Check sheet for the modelled part. Datum: model origin and axes. Units: mm. A direction names the side the tool comes from. Round coordinates to 2 decimals unless told otherwise and drop trailing zeros. Write each loop counter-clockwise with the first axis right and the second up, starting at its lowest first coordinate (ties: lowest second). Pieces come first, ordered by that corner, then holes. Notation, with made-up numbers: (-12.75, 71.25) - (10.25, 71.25) arc R12 cw to (10.25, 77.25) - close; hole circle Ø8 at (-10.75, 57.25). An arc over 180 degrees is marked (long way). Answer as a JSON object with one key per item and string values. Group by question number.
Item 1: Sectioned sample at B-B on z = 8.75. Record the boundary of the cut face in (x, y), plus the area to 3 significant figures.
Item 2: Release check for a two-part mould opening along X. For faces 1 (the cylindrical face through (-40.6, -26.43, 19.26)), 2 (the flat face through (45, 0, 10)), 3 (the cylindrical face through (-26.503, 25.131, 2.465)) record: pulls with the +X half, pulls with the -X half, needs draft (parallel to the pull), parting line crosses it, or undercut.
Item 3: Thickness scan on line 1 (Y direction, x = -24.5, z = 1.15); line 2 (X direction, y = 1.5, z = 12). Record the ranges inside material, lowest first.
Item 4: Sectioned sample at C-C on x = -20.5. Record the boundary of the cut face in (y, z).
Item 5: Set-up check for faces 4 (the cylindrical face through (26.43, -40.6, 19.26)), 5 (the flat face through (-43, 22, 18.5)), 6 (the cylindrical face through (40.6, -17.57, 19.26)), 7 (the cylindrical face through (-35.521, 38.966, 10.14)), 8 (the flat face through (-30, 0, 12)): record each of +Z, -Z, +X, -X, +Y, -Y from which the full face is reachable in a straight line by a thin tool's end or side.
Item 6: Gauge pin test, flat ends, axial feed: P1, Ø0.6, axis at x = -39, z = 20, coming from the +Y side; P2, Ø1.2, axis at x = -44, z = 19.5, coming from the -Y side; P3, Ø6.5, axis at x = -24.5, y = 24.5, coming from the +Z side. Record the tip position at first contact, or that the pin passes through.
Item 7: Sectioned sample at D-D on y = -36.5. Record the boundary of the cut face in (x, z), plus the area to 3 significant figures.
Item 8: Sectioned sample at A-A on y = 10.5. Record the boundary of the cut face in (x, z), plus the area to 3 significant figures.
```python
from build123d import *

# Parameters (mm, degrees)
ESQUISSE1_W             = 90
ESQUISSE1_H             = 90
BOSS_EXTRU_1_DEPTH      = 20
ENL_V_MAT_EXTRU_1_DEPTH = 15
ENL_V_MAT_EXTRU_2_DEPTH = 0.5
CONG_1_R                = 10
ESQUISSE6_R             = 4
ENL_V_MAT_EXTRU_4_DEPTH = 21
ESQUISSE7_R             = 5
ENL_V_MAT_EXTRU_5_DEPTH = 6
ENL_V_MAT_EXTRU_6_DEPTH = 1.5
TROU_TARAUD_M51_D       = 4.2
TROU_TARAUD_M51_DEPTH   = 14
TROU_TARAUD_M51_TIP     = 1.2618073
ENL_V_MAT_EXTRU_7_REACH = 92
ESQUISSE4_R             = 7.75


with BuildPart() as part:
    # Esquisse1 → Boss.-Extru.1 (new body)
    with BuildSketch(Plane.XY):
        Rectangle(ESQUISSE1_W, ESQUISSE1_H)
    extrude(amount=BOSS_EXTRU_1_DEPTH)

    # Esquisse2 → Enlèv. mat.-Extru.1 (cut)
    with BuildSketch(Plane.XY.offset(20)):
        with BuildLine():
            Line((-25, -30), (25, -30))
            ThreePointArc((25, -30), (28.535533906, -28.535533906), (30, -25))
            Line((30, -25), (30, 25))
            ThreePointArc((30, 25), (28.535533906, 28.535533906), (25, 30))
            Line((25, 30), (-25, 30))
            ThreePointArc((-25, 30), (-28.535533906, 28.535533906), (-30, 25))
            Line((-30, 25), (-30, -25))
            ThreePointArc((-30, -25), (-28.535533906, -28.535533906), (-25, -30))
        make_face()
    extrude(amount=-ENL_V_MAT_EXTRU_1_DEPTH, mode=Mode.SUBTRACT)

    # Esquisse3 → Enlèv. mat.-Extru.2 (cut)
    with BuildSketch(Plane.XY.offset(20)):
        with BuildLine():
            Line((25, 32), (12, 32))
            ThreePointArc((12, 32), (10.585786438, 31.414213562), (10, 30))
            Line((10, 30), (25, 30))
            ThreePointArc((25, 30), (28.535533906, 28.535533906), (30, 25))
            Line((30, 25), (30, -25))
            ThreePointArc((30, -25), (28.535533906, -28.535533906), (25, -30))
            Line((25, -30), (-25, -30))
            ThreePointArc((-25, -30), (-28.535533906, -28.535533906), (-30, -25))
            Line((-30, -25), (-30, 25))
            ThreePointArc((-30, 25), (-28.535533906, 28.535533906), (-25, 30))
            Line((-25, 30), (-10, 30))
            ThreePointArc((-10, 30), (-10.585786437, 31.414213561), (-11.999999997, 32))
            Line((-11.999999997, 32), (-25, 32))
            ThreePointArc((-25, 32), (-29.949747468, 29.949747468), (-32, 25))
            Line((-32, 25), (-32, 1))
            Line((-32, 1), (-45, 1))
            Line((-45, 1), (-45, -1))
            Line((-45, -1), (-32, -1))
            Line((-32, -1), (-32, -25))
            ThreePointArc((-32, -25), (-29.949747468, -29.949747468), (-25, -32))
            Line((-25, -32), (-1, -32))
            Line((-1, -32), (-1, -45))
            Line((-1, -45), (1, -45))
            Line((1, -45), (1, -32))
            Line((1, -32), (25, -32))
            ThreePointArc((25, -32), (29.949747468, -29.949747468), (32, -25))
            Line((32, -25), (32, -1))
            Line((32, -1), (45, -1))
            Line((45, -1), (45, 1))
            Line((45, 1), (32, 1))
            Line((32, 1), (32, 25))
            ThreePointArc((32, 25), (29.949747468, 29.949747468), (25, 32))
        make_face()
    extrude(amount=-ENL_V_MAT_EXTRU_2_DEPTH, mode=Mode.SUBTRACT)

    # Congé1
    cong_1_edges = [part.edges().sort_by_distance(p)[0] for p in [
        (45, -45, 10),
        (-45, -45, 10),
        (-45, 45, 10),
        (45, 45, 10),
    ]]
    fillet(cong_1_edges, radius=CONG_1_R)

    # Esquisse6 → Enlèv. mat.-Extru.4 (cut, through all)
    with BuildSketch(Plane.XY.offset(20)):
        with Locations((-35, 35)):
            Circle(ESQUISSE6_R)
        with Locations((35, -35)):
            Circle(ESQUISSE6_R)
    extrude(amount=-ENL_V_MAT_EXTRU_4_DEPTH, mode=Mode.SUBTRACT)

    # Esquisse7 → Enlèv. mat.-Extru.5 (cut, through all)
    with BuildSketch(Plane.XY.offset(5)):
        Circle(ESQUISSE7_R)
    extrude(amount=-ENL_V_MAT_EXTRU_5_DEPTH, mode=Mode.SUBTRACT)

    # Esquisse8 → Enlèv. mat.-Extru.6 (cut)
    with BuildSketch(Plane.XY.offset(20)):
        with BuildLine():
            Line((-27, 45), (-17, 45))
            Line((-17, 45), (-17, 42))
            ThreePointArc((-17, 42), (-17.585786438, 40.585786438), (-19, 40))
            Line((-19, 40), (-25, 40))
            ThreePointArc((-25, 40), (-26.414213562, 40.585786438), (-27, 42))
            Line((-27, 42), (-27, 45))
        make_face()
        with BuildLine():
            Line((17, 45), (27, 45))
            Line((27, 45), (27, 42))
            ThreePointArc((27, 42), (26.414213562, 40.585786438), (25, 40))
            Line((25, 40), (19, 40))
            ThreePointArc((19, 40), (17.585786438, 40.585786438), (17, 42))
            Line((17, 42), (17, 45))
        make_face()
        with BuildLine():
            Line((45, 27), (42, 27))
            ThreePointArc((42, 27), (40.585786438, 26.414213562), (40, 25))
            Line((40, 25), (40, 19))
            ThreePointArc((40, 19), (40.585786438, 17.585786438), (42, 17))
            Line((42, 17), (45, 17))
            Line((45, 17), (45, 27))
        make_face()
        with BuildLine():
            Line((45, -17), (42, -17))
            ThreePointArc((42, -17), (40.585786438, -17.585786438), (40, -19))
            Line((40, -19), (40, -25))
            ThreePointArc((40, -25), (40.585786438, -26.414213562), (42, -27))
            Line((42, -27), (45, -27))
            Line((45, -27), (45, -17))
        make_face()
        with BuildLine():
            Line((27, -45), (27, -42))
            ThreePointArc((27, -42), (26.414213562, -40.585786438), (25, -40))
            Line((25, -40), (19, -40))
            ThreePointArc((19, -40), (17.585786438, -40.585786438), (17, -42))
            Line((17, -42), (17, -45))
            Line((17, -45), (27, -45))
        make_face()
        with BuildLine():
            Line((-17, -45), (-17, -42))
            ThreePointArc((-17, -42), (-17.585786438, -40.585786438), (-19, -40))
            Line((-19, -40), (-25, -40))
            ThreePointArc((-25, -40), (-26.414213562, -40.585786438), (-27, -42))
            Line((-27, -42), (-27, -45))
            Line((-27, -45), (-17, -45))
        make_face()
        with BuildLine():
            Line((-45, -27), (-42, -27))
            ThreePointArc((-42, -27), (-40.585786438, -26.414213562), (-40, -25))
            Line((-40, -25), (-40, -19))
            ThreePointArc((-40, -19), (-40.585786438, -17.585786438), (-42, -17))
            Line((-42, -17), (-45, -17))
            Line((-45, -17), (-45, -27))
        make_face()
        with BuildLine():
            Line((-45, 17), (-42, 17))
            ThreePointArc((-42, 17), (-40.585786438, 17.585786438), (-40, 19))
            Line((-40, 19), (-40, 25))
            ThreePointArc((-40, 25), (-40.585786438, 26.414213562), (-42, 27))
            Line((-42, 27), (-45, 27))
            Line((-45, 27), (-45, 17))
        make_face()
    extrude(amount=-ENL_V_MAT_EXTRU_6_DEPTH, mode=Mode.SUBTRACT)

    # Trou taraudé M51
    with Locations(Plane(origin=(-24.5, 24.5, 5), x_dir=(1, 0, 0), z_dir=(0, 0, 1))):
        with Locations((0, 0), (49, 0), (49, -49), (0, -49)):
            Hole(TROU_TARAUD_M51_D / 2, depth=TROU_TARAUD_M51_DEPTH)
            with Locations((0, 0, -(TROU_TARAUD_M51_DEPTH + TROU_TARAUD_M51_TIP / 2))):  # 118° drill point
                Cone(0, TROU_TARAUD_M51_D / 2, TROU_TARAUD_M51_TIP, mode=Mode.SUBTRACT)

    # Esquisse4 → Enlèv. mat.-Extru.7 (cut, up to next)
    with BuildSketch(Plane(origin=(0, 45, 0), x_dir=(1, 0, 0), z_dir=(0, 1, 0)), mode=Mode.PRIVATE) as enl_v_mat_extru_7_sk1:
        with Locations((0, -20)):
            Circle(ESQUISSE4_R)
    enl_v_mat_extru_7_tool1 = extrude(enl_v_mat_extru_7_sk1.sketch, amount=-ENL_V_MAT_EXTRU_7_REACH, mode=Mode.PRIVATE) & part.part
    add(enl_v_mat_extru_7_tool1.solids().sort_by_distance((0, 45, 20))[0], mode=Mode.SUBTRACT)


solid = part.part
```
Completed:
{
 "1": {"outline": "(-45, -35) arc R10 ccw to (-35, -45) - (35, -45) arc R10 ccw to (45, -35) - (45, 35) arc R10 ccw to (35, 45) - (-35, 45) arc R10 ccw to (-45, 35) - close; hole circle Ø8 at (-35, 35); hole (-30, -25) arc R5 ccw to (-25, -30) - (25, -30) arc R5 ccw to (30, -25) - (30, 25) arc R5 ccw to (25, 30) - (-25, 30) arc R5 ccw to (-30, 25) - close; hole circle Ø8 at (35, -35)", "area": "4,340 mm²"},
 "2": {"face 1": "pulls with the -X half", "face 2": "pulls with the +X half", "face 3": "undercut"},
 "3": {"line 1": "-45 to -26.6, -22.4 to 22.4, 26.6 to 45", "line 2": "-45 to -30, 30 to 45"},
 "4": {"outline": "(-45, 0) - (45, 0) - (45, 18.5) - (40, 18.5) - (40, 20) - (32, 20) - (32, 19.5) - (30, 19.5) - (30, 5) - (-30, 5) - (-30, 19.5) - (-32, 19.5) - (-32, 20) - (-40, 20) - (-40, 18.5) - (-45, 18.5) - close"},
 "5": {"face 4": "+Z, -Y", "face 5": "+Z, -X", "face 6": "+Z, +X", "face 7": "+Z, -Z", "face 8": "+Z"},
 "6": {"P1": "y = 44.29", "P2": "y = -40.43", "P3": "z = 5"},
 "7": {"outline": "(-44.89, 0) - (31.29, 0) - (31.29, 20) - (1, 20) - (1, 19.5) - (-1, 19.5) - (-1, 20) - (-44.89, 20) - close; (38.71, 0) - (44.89, 0) - (44.89, 20) - (38.71, 20) - close", "area": "1,650 mm²"},
 "8": {"outline": "(-45, 0) - (45, 0) - (45, 20) - (32, 20) - (32, 19.5) - (30, 19.5) - (30, 5) - (-30, 5) - (-30, 19.5) - (-32, 19.5) - (-32, 20) - (-45, 20) - close", "area": "898 mm²"}
}
